from build123d import *

# Parameters (mm, degrees)
SKETCH1_R             = 14.2875
BOSS_EXTRUDE1_DEPTH   = 2.54
F_8_CLEARANCE_HOLE1_D = 4.4958


with BuildPart() as part:
    # Sketch1 → Boss-Extrude1 (new body)
    with BuildSketch(Plane(origin=(0, 0, 0), x_dir=(0, 0, -1), z_dir=(1, 0, 0))):
        with BuildLine():
            Line((57.133054897, -28.5877), (68.132491023, -28.5877))
            ThreePointArc((68.132491023, -28.5877), (74.063897019, -27.117500662), (78.622019681, -23.04729416))
            ThreePointArc((78.622019681, -23.04729416), (85.7377, 0), (78.622019681, 23.04729416))
            ThreePointArc((78.622019681, 23.04729416), (74.063897019, 27.117500662), (68.132491023, 28.5877))
            Line((68.132491023, 28.5877), (57.133054897, 28.5877))
            ThreePointArc((57.133054897, 28.5877), (49.108905845, 29.888466983), (41.906610979, 33.65754))
            ThreePointArc((41.906610979, 33.65754), (38.092212748, 34.924995225), (34.280934646, 33.648188329))
            ThreePointArc((34.280934646, 33.648188329), (20.233265061, 27.033421998), (4.712956656, 26.572790516))
            ThreePointArc((4.712956656, 26.572790516), (-26.9875, 0), (4.712956656, -26.572790516))
            ThreePointArc((4.712956656, -26.572790516), (20.233265061, -27.033421998), (34.280934646, -33.648188329))
            ThreePointArc((34.280934646, -33.648188329), (38.092212748, -34.924995225), (41.906610979, -33.65754))
            ThreePointArc((41.906610979, -33.65754), (49.108905845, -29.888466983), (57.133054897, -28.5877))
        make_face()
        Circle(SKETCH1_R, mode=Mode.SUBTRACT)
        with BuildLine():
            Line((41.2623, 19.0627), (66.6877, 19.0627))
            ThreePointArc((66.6877, 19.0627), (71.177828061, 17.202828061), (73.0377, 12.7127))
            Line((73.0377, 12.7127), (73.0377, -12.7127))
            ThreePointArc((73.0377, -12.7127), (71.177828061, -17.202828061), (66.6877, -19.0627))
            Line((66.6877, -19.0627), (41.2623, -19.0627))
            ThreePointArc((41.2623, -19.0627), (36.772171939, -17.202828061), (34.9123, -12.7127))
            Line((34.9123, -12.7127), (34.9123, 12.7127))
            ThreePointArc((34.9123, 12.7127), (36.772171939, 17.202828061), (41.2623, 19.0627))
        make_face(mode=Mode.SUBTRACT)
    extrude(amount=BOSS_EXTRUDE1_DEPTH)

    # #8 Clearance Hole1 (through all)
    with Locations(Plane(origin=(2.54, 0, 0), x_dir=(0, 0, -1), z_dir=(1, 0, 0))):
        with Locations((38.1, 28.575), (79.3877, 0), (38.1, -28.575)):
            Hole(F_8_CLEARANCE_HOLE1_D / 2)


solid = part.part
Here's how the part is built. I have some questions about the finished solid (model axes, mm). A direction names the side the tool comes from. Round coordinates to 2 decimals unless told otherwise and drop trailing zeros. Loops run counter-clockwise (first coordinate to the right, second up) from the corner with the lowest first, then second, coordinate; pieces in that order, holes last. Notation, with made-up numbers: M 19,78.25 L 57,78.25 A27 cw 57,95.25 Z; hole C 88.25,78 d6. An arc over 180 degrees is marked long. Write each question's results on one line, items separated by ' | '. Start each with the question number.
(1) I want a section at D-D (z = -38.1). Please give me the cut outline in (x, y) (3 decimals).
(2) I want a section at B-B (y = 0). Please give me the cut outline in (x, z).
(3) I want a section at A-A (z = -64). Please give me the cut outline in (x, y).
(4) On a 3-axis mill with a long thin cutter (end or side, diameter ignored), from which of +Z, -Z, +X, -X, +Y, -Y can I reach the whole of each face in a straight line? I mean faces 1 (the flat face through (1, -28.588, -63)), 2 (the cylindrical face through (1.252, -34.925, -38.035)), 3 (the cylindrical face through (1.25, -17.25, -36.82)), 4 (the flat face through (1, 28.588, -63)). Say none if no direction works.
(5) If I drill on probe 1 along Y at (x, z) = (1.3, -36.5); probe 2 along Z at (x, y) = (0.45, -11); probe 3 along Y at (x, z) = (0.8, -38.1) (3 decimals), over which ranges is the centre line in solid material (lowest first)? Write a range as from..to.
(6) Thinking about a two-plate mould opening in Y: for faces 5 (the cylindrical face through (1.25, 17.25, -71.13)), 6 (the flat face through (2.54, 0, -29)), 7 (the cylindrical face through (1.3, 27.1, -74.1)), which applies, pulls with the +Y half, pulls with the -Y half, needs draft (parallel to the pull), parting line crosses it, or undercut?
(7) I want a section at C-C (x = 0.95). State how many separate pieces and enclosed holes the cut face has, then the cut area to 3 significant figures.
(8) Will these pins go through, and if not, where does the flat tip stop? P1, Ø23, axis at y = 0, z = 0, coming from the +X side; P2, Ø2, axis at y = -18.5, z = -7.5, coming from the -X side; P3, Ø1.3, axis at x = 1.5, z = -64.5, coming from the -Y side; P4, Ø0.8, axis at x = 1.5, y = -2, coming from the +Z side.
Solved:
1) outline: M 0,-34.925 L 2.54,-34.925 L 2.54,-30.823 L 0,-30.823 Z; M 0,-26.327 L 2.54,-26.327 L 2.54,-18.219 L 0,-18.219 Z; M 0,18.219 L 2.54,18.219 L 2.54,26.327 L 0,26.327 Z; M 0,30.823 L 2.54,30.823 L 2.54,34.925 L 0,34.925 Z
2) outline: M 0,-85.74 L 2.54,-85.74 L 2.54,-81.64 L 0,-81.64 Z; M 0,-77.14 L 2.54,-77.14 L 2.54,-73.04 L 0,-73.04 Z; M 0,-34.91 L 2.54,-34.91 L 2.54,-14.29 L 0,-14.29 Z; M 0,14.29 L 2.54,14.29 L 2.54,26.99 L 0,26.99 Z
3) outline: M 0,-28.59 L 2.54,-28.59 L 2.54,-19.06 L 0,-19.06 Z; M 0,19.06 L 2.54,19.06 L 2.54,28.59 L 0,28.59 Z
4) face 1: -Z, +X, -X, -Y | face 2: +X, -X, -Y | face 3: +X, -X | face 4: -Z, +X, -X, +Y
5) probe 1: y = -34.72..-30.15, -27..-16.91, 16.91..27, 30.15..34.72 | probe 2: z = -84.23..-73.04, -34.91..-9.12, 9.12..24.64 | probe 3: y = -34.925..-30.823, -26.327..-18.219, 18.219..26.327, 30.823..34.925
6) face 5: undercut | face 6: needs draft | face 7: pulls with the +Y half
7) separate pieces: 1 | enclosed holes: 5 | area: 3,800 mm²
8) P1: passes through | P2: stops at x = 0 | P3: stops at y = -28.59 | P4: stops at z = 26.94
